Could you check a few things on this model? Use its own coordinates, in mm. A direction names the side the tool comes from. Round coordinates to 2 decimals unless told otherwise and drop trailing zeros. Loops run counter-clockwise (first coordinate to the right, second up) from the corner with the lowest first, then second, coordinate; pieces in that order, holes last. Notation, with made-up numbers: (61.5, 31.25) -> (65.5, 31.25) arc R15 ccw to (65.5, 58.25) -> close; hole circle Ø9 at (43, 24.25). An arc over 180 degrees is marked (long way). Write each question's results on one line, items separated by ' | '.
from build123d import *

# Parameters (mm, degrees)
CYLINDER009_R     = 1.8
CYLINDER009_DEPTH = 16
ARRAY009_X_COUNT  = 2
ARRAY009_X_PITCH  = 40
CYLINDER010_R     = 1.8
CYLINDER010_DEPTH = 20
ARRAY010_X_COUNT  = 2
ARRAY010_X_PITCH  = 80
ARRAY010_Z_COUNT  = 2
ARRAY010_Z_PITCH  = 43
CYLINDER011_R     = 1.8
CYLINDER011_DEPTH = 10
ARRAY011_X_COUNT  = 2
ARRAY011_X_PITCH  = 68
PAD005_DEPTH      = 10
CYLINDER008_R     = 1.8
CYLINDER008_DEPTH = 20
ARRAY008_X_COUNT  = 2
ARRAY008_X_PITCH  = 80
ARRAY008_Y_COUNT  = 2
ARRAY008_Y_PITCH  = 25
BOX005_W          = 2
BOX005_H          = 37.3
BOX005_DEPTH      = 61.3
BOX007_W          = 84.6
BOX007_H          = 2
BOX007_DEPTH      = 63.3
BOX006_W          = 84.6
BOX006_H          = 37.3
BOX006_DEPTH      = 2
BOX004_W          = 2
BOX004_H          = 37.3
BOX004_DEPTH      = 61.3
FILLET_R          = 1


with BuildPart() as cover_bottom_hole_array:
    # Cylinder009 → Cylinder009 (new body)
    with BuildSketch(Plane(origin=(20, 45, 3), x_dir=(1, 0, 0), z_dir=(0, -1, 0))):
        Circle(CYLINDER009_R)
    extrude(amount=CYLINDER009_DEPTH)

    # Array009 X: cover bottom hole array ×2


with BuildPart() as cover_bottom_hole_array_1:
    add(cover_bottom_hole_array.part)
    with Locations(*[(i * ARRAY009_X_PITCH, 0, 0) for i in range(1, ARRAY009_X_COUNT)]):
        add(cover_bottom_hole_array.part)


with BuildPart() as cover_bottom_hole_array_2:
    # Array009 placement: moved
    add(cover_bottom_hole_array_1.part.moved(Location((-40, 0, 0))))


with BuildPart() as cover_side_holes_array:
    # Cylinder010 → Cylinder010 (new body)
    with BuildSketch(Plane(origin=(-50, 3, 6), x_dir=(0, 0, -1), z_dir=(1, 0, 0))):
        Circle(CYLINDER010_R)
    extrude(amount=CYLINDER010_DEPTH)

    # Array010 X: cover side holes array ×2


with BuildPart() as cover_side_holes_array_1:
    add(cover_side_holes_array.part)
    with Locations(*[(i * ARRAY010_X_PITCH, 0, 0) for i in range(1, ARRAY010_X_COUNT)]):
        add(cover_side_holes_array.part)

    # Array010 Z: cover side holes array ×2


with BuildPart() as cover_side_holes_array_2:
    add(cover_side_holes_array_1.part)
    with Locations(*[(0, 0, i * ARRAY010_Z_PITCH) for i in range(1, ARRAY010_Z_COUNT)]):
        add(cover_side_holes_array_1.part)


with BuildPart() as cover_side_holes_array_3:
    # Array010 placement: moved
    add(cover_side_holes_array_2.part.moved(Location((0, 0, 6))))


with BuildPart() as cover_vertical_hole_array:
    # Cylinder011 → Cylinder011 (new body)
    with BuildSketch(Plane(origin=(6, 0, 50), x_dir=(1, 0, 0), z_dir=(0, 0, 1))):
        Circle(CYLINDER011_R)
    extrude(amount=CYLINDER011_DEPTH)

    # Array011 X: cover vertical hole array ×2


with BuildPart() as cover_vertical_hole_array_1:
    add(cover_vertical_hole_array.part)
    with Locations(*[(i * ARRAY011_X_PITCH, 0, 0) for i in range(1, ARRAY011_X_COUNT)]):
        add(cover_vertical_hole_array.part)


with BuildPart() as cover_vertical_hole_array_2:
    # Array011 placement: moved
    add(cover_vertical_hole_array_1.part.moved(Location((-40, 3, 6))))


with BuildPart() as wire_hole_body:
    # Sketch015 → Pad005 (new body)
    with BuildSketch(Plane.YZ.offset(42.3)):
        with BuildLine():
            Line((26, 0), (26, 13))
            ThreePointArc((26, 13), (23.5, 15.5), (21, 13))
            Line((21, 0), (21, 13))
            Line((21, 0), (26, 0))
        make_face()
    extrude(amount=-PAD005_DEPTH)


with BuildPart() as cover_extraction:
    # Cylinder008 → Cylinder008 (new body)
    with BuildSketch(Plane(origin=(-50, 6, 3), x_dir=(0, 0, -1), z_dir=(1, 0, 0))):
        Circle(CYLINDER008_R)
    extrude(amount=CYLINDER008_DEPTH)

    # Array008 X: cover extraction ×2


with BuildPart() as cover_extraction_1:
    add(cover_extraction.part)
    with Locations(*[(i * ARRAY008_X_PITCH, 0, 0) for i in range(1, ARRAY008_X_COUNT)]):
        add(cover_extraction.part)

    # Array008 Y: cover extraction ×2


with BuildPart() as cover_extraction_2:
    add(cover_extraction_1.part)
    with Locations(*[(0, i * ARRAY008_Y_PITCH, 0) for i in range(1, ARRAY008_Y_COUNT)]):
        add(cover_extraction_1.part)

    # Fusion003005: union cover bottom hole array, cover side holes array, cover vertical hole array, wire hole body
    add(cover_bottom_hole_array_2.part)
    add(cover_side_holes_array_3.part)
    add(cover_vertical_hole_array_2.part)
    add(wire_hole_body.part)


with BuildPart() as another_side_wall_cube:
    # Box005 → Box005 (new body)
    with BuildSketch(Plane(origin=(40.3, 0, 0), x_dir=(1, 0, 0), z_dir=(0, 0, 1))):
        with Locations((1, 18.65)):
            Rectangle(BOX005_W, BOX005_H)
    extrude(amount=BOX005_DEPTH)


with BuildPart() as back_cover_wall_cube:
    # Box007 → Box007 (new body)
    with BuildSketch(Plane(origin=(-42.3, 37.3, 0), x_dir=(1, 0, 0), z_dir=(0, 0, 1))):
        with Locations((42.3, 1)):
            Rectangle(BOX007_W, BOX007_H)
    extrude(amount=BOX007_DEPTH)


with BuildPart() as top_cover_wall_cube:
    # Box006 → Box006 (new body)
    with BuildSketch(Plane(origin=(-42.3, 0, 61.3), x_dir=(1, 0, 0), z_dir=(0, 0, 1))):
        with Locations((42.3, 18.65)):
            Rectangle(BOX006_W, BOX006_H)
    extrude(amount=BOX006_DEPTH)


with BuildPart() as cover_body_fillet:
    # Box004 → Box004 (new body)
    with BuildSketch(Plane(origin=(-42.3, 0, 0), x_dir=(1, 0, 0), z_dir=(0, 0, 1))):
        with Locations((1, 18.65)):
            Rectangle(BOX004_W, BOX004_H)
    extrude(amount=BOX004_DEPTH)

    # Fusion003004: union another side wall cube, back cover wall cube, top cover wall cube
    add(another_side_wall_cube.part)
    add(back_cover_wall_cube.part)
    add(top_cover_wall_cube.part)

    # Cut004: cut cover extraction
    add(cover_extraction_2.part, mode=Mode.SUBTRACT)

    # Fillet
    fillet_edges = [cover_body_fillet.edges().sort_by_distance(p)[0] for p in [
        (-42.3, 18.65, 63.3),
        (-42.3, 38.3, 63.3),
        (-42.3, 39.3, 31.65),
        (42.3, 18.65, 63.3),
        (0, 39.3, 63.3),
        (42.3, 38.3, 63.3),
        (42.3, 39.3, 31.65),
    ]]
    fillet(fillet_edges, radius=FILLET_R)


solid = cover_body_fillet.part
1) I want a section at B-B, the plane x = 34. Write out the boundary of the cut face in (y, z).
Model answer:
outline: (0, 61.3) -> (1.2, 61.3) -> (1.2, 63.3) -> (0, 63.3) -> close; (4.8, 61.3) -> (37.3, 61.3) -> (37.3, 0) -> (39.3, 0) -> (39.3, 62.3) arc R1 ccw to (38.3, 63.3) -> (4.8, 63.3) -> close
2) I want a section at A-A, the plane y = 6. Write out the boundary of the cut face in (x, z).
Model answer:
outline: (-42.3, 0) -> (-40.3, 0) -> (-40.3, 1.2) -> (-42.3, 1.2) -> close; (-42.3, 4.8) -> (-40.3, 4.8) -> (-40.3, 61.3) -> (40.3, 61.3) -> (40.3, 4.8) -> (42.3, 4.8) -> (42.3, 62.3) arc R1 ccw to (41.3, 63.3) -> (-41.3, 63.3) arc R1 ccw to (-42.3, 62.3) -> close; (40.3, 0) -> (42.3, 0) -> (42.3, 1.2) -> (40.3, 1.2) -> close
3) I want a section at C-C, the plane z = 12. Write out the boundary of the cut face in (x, y).
Model answer:
outline: (-42.3, 0) -> (-40.3, 0) -> (-40.3, 1.2) -> (-42.3, 1.2) -> close; (-42.3, 4.8) -> (-40.3, 4.8) -> (-40.3, 37.3) -> (40.3, 37.3) -> (40.3, 26) -> (42.3, 26) -> (42.3, 38.3) arc R1 ccw to (41.3, 39.3) -> (-41.3, 39.3) arc R1 ccw to (-42.3, 38.3) -> close; (40.3, 0) -> (42.3, 0) -> (42.3, 1.2) -> (40.3, 1.2) -> close; (40.3, 4.8) -> (42.3, 4.8) -> (42.3, 21) -> (40.3, 21) -> close
4) If we mould it in two halves opening along X, with no side actions, what happens to faces 1 (the cylindrical face through (-41.314, 4.785, 55.234)), 2 (the cylindrical face through (35.717, 3.541, 62.286)), 3 (the flat face through (-42.3, 19, 31)), 4 (the flat face through (-40.3, 18, 30))? For each: released by +X, released by -X, zero draft, split by the parting line, or undercut.
Model answer:
face 1: zero draft | face 2: undercut | face 3: released by -X | face 4: undercut
5) I'm going to push flat-ended pins straight in: pin 1 (6 mm diameter, centred on x = -24.5, y = 14, fed in from -Z); pin 2 (4 mm diameter, centred on x = 25, z = 56.5, fed in from -Y). Where does each tip first touch, or does it pass through?
Model answer:
pin 1: stops at z = 61.3 | pin 2: stops at y = 37.3
6) I need wall thicknesses on line 1 (Y direction, x = 41.35, z = 12); line 2 (Z direction, x = -41, y = 3); line 3 (X direction, y = 38.1, z = 3). Which ranges of each line are inside material? Lowest first, please.
Model answer:
line 1: y = 0 to 1.2, 4.8 to 21, 26 to 39.3 | line 2: z = 0 to 10.2, 13.8 to 53.2, 56.8 to 63.3 | line 3: x = -42.3 to -21.8, -18.2 to 18.2, 21.8 to 42.3
7) For faces 5 (the flat face through (41, 21, 6)), 6 (the flat face through (40.3, 18, 30)), 7 (the flat face through (-13, 39, 0)), which set-ups out of +Z, -Z, +X, -X, +Y, -Y let a thin tool reach every point of the face, with its end or its side?
Model answer:
face 5: -Z, +X | face 6: -Z, -Y | face 7: -Z, +X, -X, +Y, -Y
8) I want a section at D-D, the plane y = 10. Write out the boundary of the cut face in (x, z), plus the area to 3 significant figures.
Model answer:
outline: (-42.3, 0) -> (-40.3, 0) -> (-40.3, 61.3) -> (40.3, 61.3) -> (40.3, 0) -> (42.3, 0) -> (42.3, 62.3) arc R1 ccw to (41.3, 63.3) -> (-41.3, 63.3) arc R1 ccw to (-42.3, 62.3) -> close | area: 414 mm2
